from build123d import *

# Parameters (mm, degrees)
SKETCH_1_W          = 20
SKETCH_1_H          = 20
SKETCH_1_W_2        = 16
SKETCH_1_H_2        = 16
EXTRUDE_1_DEPTH     = 560
SKETCH_2_R          = 2.1
CUT_EXTRUDE_1_DEPTH = 10
SKETCH_4_R          = 2.2
CUT_EXTRUDE_3_DEPTH = 21
SKETCH_5_R          = 2.1
CUT_EXTRUDE_4_DEPTH = 22


with BuildPart() as part:
    # ｽｹｯﾁ1 → ﾎﾞｽ - 押し出し1 (new body)
    with BuildSketch(Plane.XY):
        Rectangle(SKETCH_1_W, SKETCH_1_H)
        Rectangle(SKETCH_1_W_2, SKETCH_1_H_2, mode=Mode.SUBTRACT)
    extrude(amount=EXTRUDE_1_DEPTH)

    # ｽｹｯﾁ2 → ｶｯﾄ - 押し出し1 (cut)
    with BuildSketch(Plane(origin=(0, 10, 0), x_dir=(1, 0, 0), z_dir=(0, 1, 0))):
        with Locations((0, -550)):
            Circle(SKETCH_2_R)
        with Locations((0, -10)):
            Circle(SKETCH_2_R)
    extrude(amount=-CUT_EXTRUDE_1_DEPTH, mode=Mode.SUBTRACT)

    # ｽｹｯﾁ4 → ｶｯﾄ - 押し出し3 (cut, through all)
    with BuildSketch(Plane(origin=(10, 0, 0), x_dir=(0, 0, -1), z_dir=(1, 0, 0))):
        with Locations((-500.38, 0)):
            Circle(SKETCH_4_R)
        with Locations((-365.38, 0)):
            Circle(SKETCH_4_R)
        with Locations((-230.38, 0)):
            Circle(SKETCH_4_R)
    extrude(amount=-CUT_EXTRUDE_3_DEPTH, mode=Mode.SUBTRACT)

    # ｽｹｯﾁ5 → ｶｯﾄ - 押し出し4 (cut)
    with BuildSketch(Plane(origin=(10, 0, 0), x_dir=(0, 0, -1), z_dir=(1, 0, 0))):
        with Locations((-130, 0)):
            Circle(SKETCH_5_R)
        with Locations((-45, 0)):
            Circle(SKETCH_5_R)
    extrude(amount=-CUT_EXTRUDE_4_DEPTH, mode=Mode.SUBTRACT)


solid = part.part
For this review, take the finished solid that the model builds, in its own axes (mm). A direction names the side the tool comes from. Coordinates: 2 decimals unless noted, no trailing zeros. Write each loop counter-clockwise with the first axis right and the second up, starting at its lowest first coordinate (ties: lowest second). Pieces come first, ordered by that corner, then holes. Notation, with made-up numbers: (25.5, 58.5) -> (82.5, 58.5) arc R16 ccw to (82.5, 73.5) -> close; hole circle Ø5 at (79.25, 50). An arc over 180 degrees is marked (long way). Write each question's results on one line, items separated by ' | '. Start each with the question number.
1) Consider section A-A (z = 193). Write out the cut boundary in (x, y), plus the area to 3 significant figures.
2) For faces 1 (the face through (-8, 0, 276)), 2 (the face through (-9, 0, 560)), list the 3-axis set-ups (+Z, -Z, +X, -X, +Y, -Y) from which the entire face can be reached by the end or side of a thin tool; tool diameter is ignored.
3) Insertion check: pin 1 (3.5 mm diameter, centred on y = 0, z = 130, fed in from -X). The pin has a flat end and moves straight along its axis. Give the tip position at first contact, or say it passes through.
4) The part is to be moulded in two halves that separate along X. For faces 3 (the face through (-9, 0, 0)), 4 (the face through (10, 0, 276)), 5 (the face through (0, 8, 276)), say which applies: +X half, -X half, draft (parallel to the pull), parting line (faces both ways), or undercut.
5) Wall thickness on L1, parallel to Y at x = -5.25, z = 387; L2, parallel to Y at x = 9.1, z = 130: over which ranges is each line inside the solid? List them lowest first. Write a range as [from, to].
Geometry says:
1) outline: (-10, -10) -> (10, -10) -> (10, 10) -> (-10, 10) -> close; hole (-8, -8) -> (8, -8) -> (8, 8) -> (-8, 8) -> close | area: 144 mm^2
2) face 1: +Z, -Z | face 2: +Z, +X, -X, +Y, -Y
3) pin 1: through
4) face 3: draft | face 4: +X half | face 5: undercut
5) L1: [-10, -8], [8, 10] | L2: [-10, -2.1], [2.1, 10]
